Autodesk Inventor part; units mm, degrees
ref_plane "YZ Plane" through (0, 0, 0) normal (1, 0, 0) x (0, 1, 0)
ref_plane "XZ Plane" through (0, 0, 0) normal (0, 1, 0) x (-1, 0, 0)
ref_plane "XY Plane" through (0, 0, 0) normal (0, 0, 1) x (1, 0, 0)
sketch "Sketch1" plane through (0, 0, 0) normal (0, 0, 1) x (1, 0, 0)
  line L0 (0, 0) -> (123, 0)
  line L1 (123, 0) -> (123, 79)
  line L2 (123, 79) -> (0, 79)
  line L3 (0, 79) -> (0, 0)
  line L4 (12, 79) -> (12, 0)
  line L5 (123, 69.5) -> (126.5, 69.5)
  line L6 (126.5, 69.5) -> (126.5, 9.5)
  line L7 (126.5, 9.5) -> (123, 9.5)
  line L8 (123, 9.5) -> (123, 69.5)
  line L9 (126.5, 9.5) -> (132.5, 9.5)
  line L10 (132.5, 9.5) -> (132.5, 69.5)
  line L11 (132.5, 69.5) -> (126.5, 69.5)
  line L12 (126.5, 69.5) -> (126.5, 9.5)
  line L13 (123, 69.5) -> (119, 69.5)
  line L14 (119, 69.5) -> (119, 79)
  line L15 (119, 79) -> (123, 79)
  line L16 (123, 79) -> (123, 69.5)
  line L17 (123, 9.5) -> (119, 9.5)
  line L18 (119, 9.5) -> (119, 0)
  line L19 (119, 0) -> (123, 0)
  line L20 (123, 0) -> (123, 9.5)
  circle A0 centre (129.5, 39.5) radius 2.1
  line L21 (9, 39.5) -> (5, 39.5) construction
  line L22 (9, 42) -> (5, 42)
  line L23 (5, 37) -> (9, 37)
  arc A1 (9, 37) -> (9, 42) centre (9, 39.5) ccw
  arc A2 (5, 42) -> (5, 37) centre (5, 39.5) ccw
  point P0 (7, 39.5)
  dimension "d0" = 123
  dimension "d1" = 79
  dimension "d2" = 111
  dimension "d3" = 3.5
  dimension "d4" = 6
  dimension "d5" = 60
  dimension "d6" = 9.5
  dimension "d7" = 4
  dimension "d8" = 4
  dimension "d9" = 4.2
  dimension "d10" = 3
  dimension "d11" = 30
  dimension "d20" = 5
  dimension "d21" = 3
  dimension "d22" = 4
  dimension "d23" = 39.5
extrude "Extrusion1" add sketch "Sketch1" along normal blind 2 contours L3 L2 L4 L0 | L4 L2 L14 L13 L1 L17 L18 L0 | L1 L5 L6 L7 | L6 L11 L10 L9 | A0
extrude "Extrusion3" add sketch "Sketch1" against normal blind 2 contours L4 L2 L14 L13 L1 L17 L18 L0 | L6 L11 L10 L9
sketch "Sketch2" plane through (0, 0, 2) normal (0, 0, 1) x (1, 0, 0)
  circle A0 centre (60, 39.5) radius 34
  line L0 (119, 79) -> (0, 79)
  line L1 (0, 79) -> (0, 0)
  line L2 (59, 52.5) -> (64, 52.5)
  line L3 (64, 52.5) -> (64, 47.5)
  line L4 (64, 47.5) -> (59, 47.5)
  line L5 (59, 47.5) -> (59, 52.5)
  line L6 (59, 31.5) -> (64, 31.5)
  line L7 (64, 31.5) -> (64, 26.5)
  line L8 (64, 26.5) -> (59, 26.5)
  line L9 (59, 26.5) -> (59, 31.5)
  circle A1 centre (33, 39.5) radius 1.5
  circle A2 centre (33, 39.5) radius 4
  line L10 (35, 42.9641) -> (35, 36.0359)
  line L11 (33, 41) -> (35, 41)
  line L12 (33, 38) -> (35, 38)
  circle A3 centre (33, 39.5) radius 5
  line L13 (35, 42.9641) -> (35, 44.0826)
  line L14 (35, 36.0359) -> (35, 34.9174)
  line L15 (35, 42.9641) -> (49, 42.9641)
  line L16 (49, 42.9641) -> (49, 36.0359)
  line L17 (49, 36.0359) -> (35, 36.0359)
  line L18 (35, 36.0359) -> (35, 42.9641)
  dimension "d24" = 68
  dimension "d25" = 39.5
  dimension "d26" = 60
  dimension "d27" = 16
  dimension "d28" = 5
  dimension "d29" = 5
  dimension "d30" = 8
  dimension "d31" = 5
  dimension "d32" = 31
  dimension "d33" = 27
  dimension "d34" = 3
  dimension "d35" = 8
  dimension "d36" = 64
  dimension "d37" = 2
  dimension "d38" = 10
  dimension "d51" = 16
  dimension "d52" = 6.9282
extrude "Extrusion4" add sketch "Sketch2" along normal blind 3.7 contours L2 L3 L4 L5 | L6 L7 L8 L9
sketch "Sketch3" plane through (0, 0, 5.7) normal (0, 0, 1) x (1, 0, 0)
  line L0 (59, 52.5) -> (64, 52.5)
  line L1 (59, 52.5) -> (65.1, 52.5)
  line L2 (65.1, 52.5) -> (65.1, 47.5)
  line L3 (65.1, 47.5) -> (59, 47.5)
  line L4 (59, 47.5) -> (59, 52.5)
  line L5 (59, 47.5) -> (64, 47.5)
  line L6 (59, 31.5) -> (64, 31.5)
  line L7 (59, 31.5) -> (65.1, 31.5)
  line L8 (65.1, 31.5) -> (65.1, 26.5)
  line L9 (65.1, 26.5) -> (59, 26.5)
  line L10 (59, 26.5) -> (59, 31.5)
  line L11 (59, 26.5) -> (64, 26.5)
  line L12 (64, 47.5) -> (64, 52.5)
  line L13 (64, 26.5) -> (64, 31.5)
  point P0 (0, 0)
  point P1 (61.5, 47.5)
  point P2 (61.5, 26.5)
  dimension "d41" = 1.1
  dimension "d42" = 1.1
extrude "Extrusion5" add sketch "Sketch3" against normal blind 1.3
fillet "Fillet1" radius 0.25 4 edges at (59, 29, 5.7) (59, 50, 5.7) (64, 29, 4.4) (64, 50, 4.4)
extrude "Extrusion6" add sketch "Sketch2" along normal blind 4.5 contours A2 L14 A3 L13
sketch "Sketch4" plane through (0, 0, 6.5) normal (0, 0, 1) x (1, 0, 0)
  line L0 (35, 42.9641) -> (35, 36.0359)
  line L1 (33, 41) -> (35, 41)
  circle A0 centre (33, 39.5) radius 1.5
  line L2 (33, 38) -> (35, 38)
  arc A1 (35, 42.9641) -> (35, 36.0359) centre (33, 39.5) ccw
  point P0 (0, 0)
extrude "Extrusion7" add sketch "Sketch4" against normal blind 2 contours L0 L1 A0 L2 A1
fillet "Fillet2" radius 1 2 edges at (35, 36.4587, 6.5) (35, 42.5413, 6.5)
extrude "Extrusion8" cut sketch "Sketch2" against normal through all contours A1 | A1 L11 L10 L12 | A1 L12 L10 A2 L11 | L10 A2 | L15 A3 L17 A2 | L15 L16 L17 A3
fillet "Fillet3" radius 1 5 edges at (34.7352, 34.8107, 6.1779) (35, 34.9174, 3.75) (34.7352, 44.1893, 6.1779) (35, 44.0826, 3.75) (28, 39.5, 6.5)
sketch "Sketch5" plane through (0, 0, 2) normal (0, 0, 1) x (1, 0, 0)
  point P0 (0, 0)
extrude "Extrusion9" cut sketch "Sketch1" along normal through all both and the other way through all contours A0
equation "\"d6\" = -0.5 * d5 + 0.5 * d1"
equation "\"d10\" = 0.5 * d4"
equation "\"d11\" = 0.5 * d5"
equation "\"d25\" = d23"
equation "\"d29\" = d28"
equation "\"d30\" = 0.5 * d27"
properties part number "gps_cover"
The listing builds one solid part. Answer for the finished solid, in the listing's coordinates (mm). A direction names the side the tool comes from. Give positions to 0.01 mm unless a question says otherwise; leave off trailing zeros. Write each loop counter-clockwise with the first axis right and the second up, starting at its lowest first coordinate (ties: lowest second). Pieces come first, ordered by that corner, then holes. Notation, with made-up numbers: (-4, 61) -> (52, 61) arc R11 cw to (52, 67) -> close; hole circle Ø3 at (-36.5, 58.25). An arc over 180 degrees is marked (long way). Write item = value, one per line. Start each with the question number.
1) The part is cut by section A-A, the plane x = 129.5. Determine the outline of the cut face in (y, z).
2) Straight lines are drawn through the part: line 1 along X through (y, z) = (14, -0.25); line 2 along Y through (x, z) = (129.5, -0.1); line 3 along Y through (x, z) = (33, 1.5). For each, find the intervals that lie inside material, in ascending order.
3) The part is cut by section B-B, the plane y = 39.5. Determine the outline of the cut face in (x, z), and give its area (3 significant figures).
4) Determine the mould class of faces 1 (the face through (61, 26.5, 4)), 2 (the face through (35, 42, 5)), 3 (the face through (11.5, 39.6, 1)) for opening direction Y: +Y half, -Y half, draft (parallel to the pull), parting line (faces both ways), or undercut.
5) The part is cut by section C-C, the plane x = 107. Determine the outline of the cut face in (y, z).
6) Each of these flat-tipped pins is pushed along its axis until it touches: pin 1 (1.8 mm diameter, centred on x = 61, z = 3.5, fed in from -Y); pin 2 (6.5 mm diameter, centred on x = 33, y = 39.5, fed in from -Z); pin 3 (8 mm diameter, centred on x = 72, y = 37, fed in from +Z). Where does it stop, or does it pass through?
7) Which of the six approach directions +Z, -Z, +X, -X, +Y, -Y give full straight-line access (tool end or side, diameter ignored) to faces 4 (the face through (59, 29, 4)), 5 (the face through (42, 42.964, 0)), 6 (the face through (31, 40, 4.5))?
Solutions:
q1.outline = (9.5, -2) -> (37.4, -2) -> (37.4, 2) -> (9.5, 2) -> close; (41.6, -2) -> (69.5, -2) -> (69.5, 2) -> (41.6, 2) -> close
q2.line_1 = 12 to 123, 126.5 to 132.5
q2.line_2 = 9.5 to 37.4, 41.6 to 69.5
q2.line_3 = 0 to 35.5, 43.5 to 79
q3.outline = (0, 0) -> (2.5, 0) -> (2.5, 2) -> (0, 2) -> close; (11.5, 0) -> (12, 0) -> (12, -2) -> (29, -2) -> (29, 4.5) -> (31.5, 4.5) -> (31.5, 6.5) -> (29, 6.5) arc R1 ccw to (28, 5.5) -> (28, 2) -> (11.5, 2) -> close; (49, -2) -> (123, -2) -> (123, 0) -> (126.5, 0) -> (126.5, -2) -> (127.4, -2) -> (127.4, 2) -> (49, 2) -> close; (131.6, -2) -> (132.5, -2) -> (132.5, 2) -> (131.6, 2) -> close
q3.area = 393 mm²
q4.face_1 = -Y half
q4.face_2 = draft
q4.face_3 = undercut
q5.outline = (0, -2) -> (79, -2) -> (79, 2) -> (0, 2) -> close
q6.pin_1 = 26.5
q6.pin_2 = 4.5
q6.pin_3 = 2
q7.face_4 = +Z, -X, +Y, -Y
q7.face_5 = +Z, -Z
q7.face_6 = -Z
